Work out the finished part from the listing and answer in its coordinate system (mm). Face numbers are marked on the shaded views. A direction names the side the tool comes from. Coordinates: 2 decimals unless noted, no trailing zeros. Order: outer loops, then holes, each group sorted by start corner. A loop starts at its lowest first (then second) coordinate and runs counter-clockwise, first axis right, second up. Notation, with made-up numbers: (66, 27.5) -> (123, 27.5) arc R25 cw to (123, 54.5) -> close; hole circle Ø5 at (81.25, -32.75). An arc over 180 degrees is marked (long way). Answer as CSV lines item,"result". Start each with the question number.
Item 1: A straight line is drawn through the part: L1, parallel to X at y = -59, z = 8.5. Find the intervals that lie inside material, in ascending order.
Item 2: Section A-A (z = -4) is taken. Write down the section's boundary in (x, y).
Item 3: Section B-B (x = 15) is taken. Write down the section's boundary in (y, z), then the cut area to 3 significant figures.
Item 4: Each of these flat-tipped pins is pushed along its axis until it touches: pin 1 Ø12 at (x, z) = (26.5, 1) entering from -Y; pin 2 Ø4 at (x, y) = (10.5, -54) entering from +Z; pin 3 Ø1 at (x, z) = (-24.5, -5) entering from +Y. Where does it stop, or does it pass through?
Item 5: Which of the six approach directions +Z, -Z, +X, -X, +Y, -Y give full straight-line access (tool end or side, diameter ignored) to the marked faces 1 and 2?
```python
from build123d import *

# Parameters (mm, degrees)
F0_W      = 101.6
F0_H      = 38.1
F1_DEPTH  = 25.4
F2_W      = 50.8
F2_H      = 38.1
F3_DEPTH  = 25.4
F1_FACE_W = 50.8
F1_FACE_H = 38.1
F4_DEPTH  = 50.8


with BuildPart() as f1:
    # F0 (on Front) → F1 (new body)
    with BuildSketch(Plane.XZ):
        Rectangle(F0_W, F0_H)
    extrude(amount=F1_DEPTH)

    # F2 (on face) → F3 (join)
    with BuildSketch(Plane.XZ.offset(25.4)):
        with Locations((25.4, 0)):
            Rectangle(F2_W, F2_H)
    extrude(amount=F3_DEPTH)

    # F1_face (on face) → F4 (join)
    with BuildSketch(Plane.XZ.offset(25.4)):
        with Locations((-25.4, 0)):
            Rectangle(F1_FACE_W, F1_FACE_H)
    extrude(amount=F4_DEPTH)


solid = f1.part
```
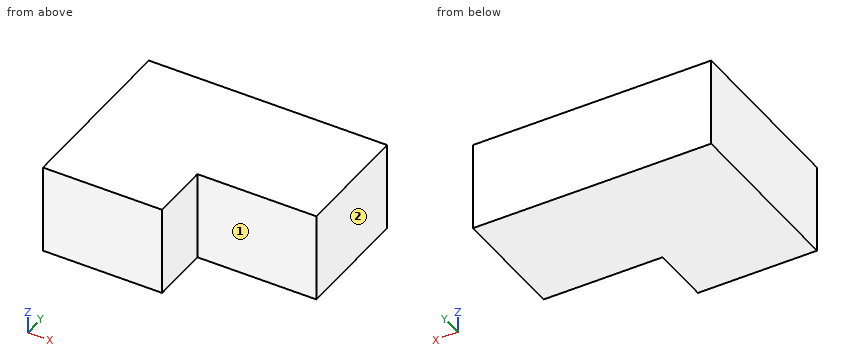
Checked values:
1,L1,"x = -50.8 to 0"
2,outline,"(-50.8, -76.2) -> (0, -76.2) -> (0, -50.8) -> (50.8, -50.8) -> (50.8, 0) -> (-50.8, 0) -> close"
3,outline,"(-50.8, -19.05) -> (0, -19.05) -> (0, 19.05) -> (-50.8, 19.05) -> close"
3,area,"1,940 mm^2"
4,pin 1,"stops at y = -50.8"
4,pin 2,"passes through"
4,pin 3,"stops at y = 0"
5,face 1,"+Z, -Z, +X, -Y"
5,face 2,"+Z, -Z, +X, +Y, -Y"
